Can you work these out from the model? Positions are in its coordinate system, mm. Face numbers are marked on the shaded views. A direction names the side the tool comes from. Give positions to 0.01 mm unless a question says otherwise; leave off trailing zeros. Order: outer loops, then holes, each group sorted by start corner. A loop starts at its lowest first (then second) coordinate and runs counter-clockwise, first axis right, second up. Notation, with made-up numbers: (-5.75, 34) - (27.25, 34) arc R10 ccw to (27.25, 52) - close; hole circle Ø8 at (11.5, 25.5). An arc over 180 degrees is marked (long way). Write each question's results on one line, items separated by ' | '. Start each with the question number.
from build123d import *

# Parameters (mm, degrees)
F0_R     = 1.5
F1_DEPTH = 5
F2_R     = 1.75
F4_DEPTH = 7
F3_W     = 5
F3_H     = 31
F5_DEPTH = 20
F6_R     = 1.5
F7_DEPTH = 25


with BuildPart() as f1:
    # F0 (on Top) → F1 (new body)
    with BuildSketch(Plane.XY):
        Polygon((24, 0), (0, 0), (0, -31), (5, -31), (5, -5), (24, -5), align=None)
        with Locations((8.085881, -2.5)):
            Circle(F0_R, mode=Mode.SUBTRACT)
    extrude(amount=F1_DEPTH)

    # F2 (on Top) → F4 (cut)
    with BuildSketch(Plane.XY):
        with Locations((21.5, -2.5)):
            Circle(F2_R)
    extrude(amount=F4_DEPTH, mode=Mode.SUBTRACT)

    # F3 (on face) → F5 (join)
    with BuildSketch(Plane.XY.offset(5)):
        with Locations((2.5, -15.5)):
            Rectangle(F3_W, F3_H)
    extrude(amount=-F5_DEPTH)

    # F6 (on face) → F7 (cut)
    with BuildSketch(Plane(origin=(0, 0, 0), x_dir=(0, -1, 0), z_dir=(-1, 0, 0))):
        with Locations((23, -12.5)):
            Circle(F6_R)
        with Locations((4, -12.5)):
            Circle(F6_R)
    extrude(amount=-F7_DEPTH, mode=Mode.SUBTRACT)


solid = f1.part
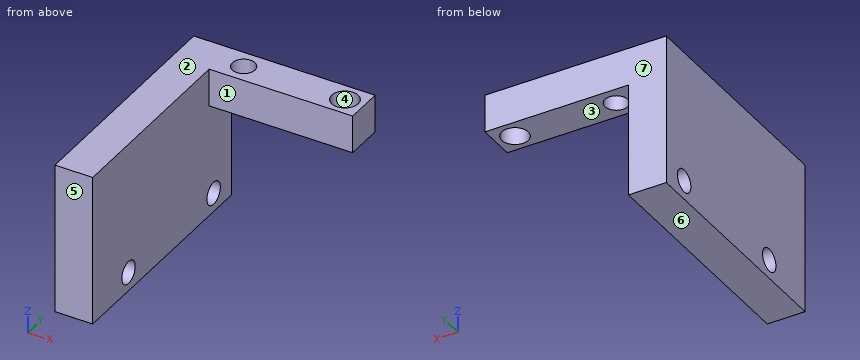
Q1. If we section it at C-C (x = 21.5): Please give me the cut outline in (y, z), plus the area to 3 significant figures.
Q2. If we section it at B-B (z = -12.5): Please give me the cut outline in (x, y), plus the area to 3 significant figures.
Q3. If we section it at A-A (y = -23): Please give me the cut outline in (x, z).
Q4. If we section it at D-D (z = 3.75): Please give me the cut outline in (x, y).
Q5. If I drill on probe 1 along Y at (x, z) = (21.5, 2.1); probe 2 along X at (y, z) = (-19.5, -8.5); probe 3 along Z at (x, y) = (3.4, -4), over which ranges is the centre line in solid material (lowest first)? Write a range as from..to.
Q6. Thinking about a two-plate mould opening in Y: for the marked faces 4, 5, 6 and 7, which applies, released by +Y, released by -Y, zero draft, split by the parting line, or undercut?
Q7. Will these pins go through, and if not, where does the flat tip stop? P1, Ø5, axis at y = -4, z = -12.5, coming from the +X side; P2, Ø1.8, axis at y = -23, z = -12.5, coming from the +X side; P3, Ø5.5, axis at x = 21.5, y = -2.5, coming from the -Z side; P4, Ø1.5, axis at x = 12, z = 2, coming from the -Y side.
Q8. Which directions (+Z, -Z, +X, -X, +Y, -Y) give clear straight access to the entire face, cutting with the end or side of a thin tool? Please do the marked faces 1, 2 and 3.
Findings below:
1) outline: (-5, 0) - (-4.25, 0) - (-4.25, 5) - (-5, 5) - close; (-0.75, 0) - (0, 0) - (0, 5) - (-0.75, 5) - close | area: 7.50 mm2
2) outline: (0, -31) - (5, -31) - (5, -24.5) - (0, -24.5) - close; (0, -21.5) - (5, -21.5) - (5, -5.5) - (0, -5.5) - close; (0, -2.5) - (5, -2.5) - (5, 0) - (0, 0) - close | area: 125 mm2
3) outline: (0, -15) - (5, -15) - (5, -14) - (0, -14) - close; (0, -11) - (5, -11) - (5, 5) - (0, 5) - close
4) outline: (0, -31) - (5, -31) - (5, -5) - (24, -5) - (24, 0) - (0, 0) - close; hole circle Ø3 at (8.09, -2.5); hole circle Ø3.5 at (21.5, -2.5)
5) probe 1: y = -5..-4.25, -0.75..0 | probe 2: x = 0..5 | probe 3: z = -15..-14, -11..5
6) face 4: undercut | face 5: released by -Y | face 6: zero draft | face 7: released by +Y
7) P1: stops at x = 5 | P2: passes through | P3: stops at z = 0 | P4: stops at y = -5
8) face 1: +Z, -Z, +X, -Y | face 2: +Z, +X, -X, +Y, -Y | face 3: -Z, +X, +Y, -Y
